Verification items for this drawing (mm, ordinates from the low corner). A direction names the side the tool comes from. Give positions to 0.01 mm unless a question says otherwise; leave off trailing zeros. Write each loop counter-clockwise with the first axis right and the second up, starting at its lowest first coordinate (ties: lowest second). Pieces come first, ordered by that corner, then holes. Notation, with made-up numbers: (3, 69.5) -> (43, 69.5) arc R27 cw to (43, 89.5) -> close; hole circle Ø7 at (-37, 65.5). An arc over 180 degrees is marked (long way). One line per item, written item: value.
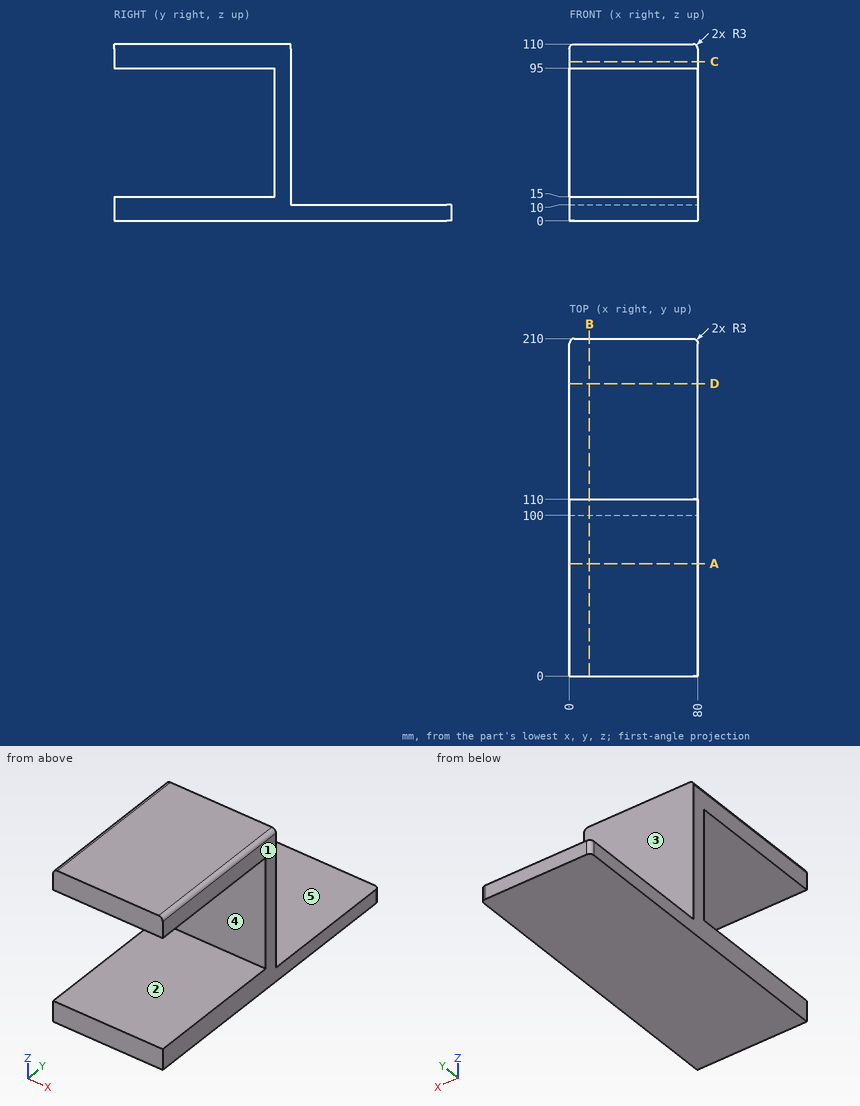
1) Mould release check, pull along Z, two halves, no side actions. Record for the marked faces 3, 4 and 5: released by +Z, released by -Z, zero draft, split by the parting line, or undercut.
Verdict:
face 3: zero draft
face 4: undercut
face 5: released by +Z
2) Depth check by flat-ended pin: pin 1 Ø12 at (x, z) = (19, 65) entering from +Y; pin 2 Ø1.5 at (x, y) = (61, 155) entering from +Z; pin 3 Ø2 at (x, z) = (68.5, 90) entering from -Y. Enter the tip coordinate at first touch or a pass-through.
Verdict:
pin 1: y = 110
pin 2: z = 10
pin 3: y = 100
3) Sectioned sample at C-C on z = 99. Record the cut outline in (x, y).
Verdict:
outline: (0, 0) -> (80, 0) -> (80, 110) -> (0, 110) -> close
4) Sectioned sample at D-D on y = 182. Record the cut outline in (x, z).
Verdict:
outline: (0, 0) -> (80, 0) -> (80, 10) -> (0, 10) -> close
5) Scan lines: probe 1 along Z at (x, y) = (54.5, 36); probe 2 along Z at (x, y) = (44, 123); probe 3 along Y at (x, z) = (52.5, 77.5). Record each from-to range of solid material in increasing order.
Verdict:
probe 1: 0 to 15, 95 to 110
probe 2: 0 to 10
probe 3: 100 to 110
6) Sectioned sample at A-A on y = 70. Record the cut outline in (x, z), plus the area to 3 significant figures.
Verdict:
outline: (0, 0) -> (80, 0) -> (80, 15) -> (0, 15) -> close; (0, 95) -> (80, 95) -> (80, 107) arc R3 ccw to (77, 110) -> (3, 110) arc R3 ccw to (0, 107) -> close
area: 2,400 mm^2
7) Tool access check on the marked faces 1 and 2. Record the directions out of +Z, -Z, +X, -X, +Y, -Y that give a thin tool (end or side, any length) a straight path to the whole face; none if there is none.
Verdict:
face 1: +Z, -Z, +X, +Y, -Y
face 2: +X, -X, -Y
8) Sectioned sample at B-B on x = 12.5. Record the cut outline in (y, z), plus the area to 3 significant figures.
Verdict:
outline: (0, 0) -> (210, 0) -> (210, 10) -> (110, 10) -> (110, 110) -> (0, 110) -> (0, 95) -> (100, 95) -> (100, 15) -> (0, 15) -> close
area: 5,100 mm^2
